from build123d import *

# Parameters (mm, degrees)
F1_DEPTH = 238.125
F3_DEPTH = 1.017


with BuildPart() as f1:
    # F0 (on Right) → F1 (new body, symmetric)
    with BuildSketch(Plane.YZ):
        Polygon((1.016, 17.526), (0, 17.526), (0, 12.446), (6.604, 12.446), (6.604, -12.446), (0, -12.446), (0, -17.526), (1.016, -17.526), (1.016, -13.462), (7.62, -13.462), (7.62, 13.462), (1.016, 13.462), align=None)
    extrude(amount=F1_DEPTH, both=True)

    # F2 (on face) → F3 (cut, through all)
    with BuildSketch(Plane.XZ.offset(-6.604)):
        with BuildLine():
            Line((-196.62013, 3.175), (-204.95387, 3.175))
            ThreePointArc((-204.95387, 3.175), (-208.12887, 0), (-204.95387, -3.175))
            Line((-204.95387, -3.175), (-196.62013, -3.175))
            ThreePointArc((-196.62013, -3.175), (-193.44513, 0), (-196.62013, 3.175))
        make_face()
        with BuildLine():
            ThreePointArc((-229.84587, 3.175), (-233.02087, 0), (-229.84587, -3.175))
            Line((-229.84587, -3.175), (-221.51213, -3.175))
            ThreePointArc((-221.51213, -3.175), (-218.33713, 0), (-221.51213, 3.175))
            Line((-221.51213, 3.175), (-229.84587, 3.175))
        make_face()
        with BuildLine():
            Line((-171.72813, 3.175), (-180.06187, 3.175))
            ThreePointArc((-180.06187, 3.175), (-183.23687, 0), (-180.06187, -3.175))
            Line((-180.06187, -3.175), (-171.72813, -3.175))
            ThreePointArc((-171.72813, -3.175), (-168.55313, 0), (-171.72813, 3.175))
        make_face()
        with BuildLine():
            Line((-146.83613, 3.175), (-155.16987, 3.175))
            ThreePointArc((-155.16987, 3.175), (-158.34487, 0), (-155.16987, -3.175))
            Line((-155.16987, -3.175), (-146.83613, -3.175))
            ThreePointArc((-146.83613, -3.175), (-143.66113, 0), (-146.83613, 3.175))
        make_face()
        with BuildLine():
            Line((-121.94413, 3.175), (-130.27787, 3.175))
            ThreePointArc((-130.27787, 3.175), (-133.45287, 0), (-130.27787, -3.175))
            Line((-130.27787, -3.175), (-121.94413, -3.175))
            ThreePointArc((-121.94413, -3.175), (-118.76913, 0), (-121.94413, 3.175))
        make_face()
        with BuildLine():
            Line((-97.05213, 3.175), (-105.38587, 3.175))
            ThreePointArc((-105.38587, 3.175), (-108.56087, 0), (-105.38587, -3.175))
            Line((-105.38587, -3.175), (-97.05213, -3.175))
            ThreePointArc((-97.05213, -3.175), (-93.87713, 0), (-97.05213, 3.175))
        make_face()
        with BuildLine():
            Line((-72.16013, 3.175), (-80.49387, 3.175))
            ThreePointArc((-80.49387, 3.175), (-83.66887, 0), (-80.49387, -3.175))
            Line((-80.49387, -3.175), (-72.16013, -3.175))
            ThreePointArc((-72.16013, -3.175), (-68.98513, 0), (-72.16013, 3.175))
        make_face()
        with BuildLine():
            Line((-47.26813, 3.175), (-55.60187, 3.175))
            ThreePointArc((-55.60187, 3.175), (-58.77687, 0), (-55.60187, -3.175))
            Line((-55.60187, -3.175), (-47.26813, -3.175))
            ThreePointArc((-47.26813, -3.175), (-44.09313, 0), (-47.26813, 3.175))
        make_face()
        with BuildLine():
            Line((-22.37613, 3.175), (-30.70987, 3.175))
            ThreePointArc((-30.70987, 3.175), (-33.88487, 0), (-30.70987, -3.175))
            Line((-30.70987, -3.175), (-22.37613, -3.175))
            ThreePointArc((-22.37613, -3.175), (-19.20113, 0), (-22.37613, 3.175))
        make_face()
        with BuildLine():
            Line((2.51587, 3.175), (-5.81787, 3.175))
            ThreePointArc((-5.81787, 3.175), (-8.99287, 0), (-5.81787, -3.175))
            Line((-5.81787, -3.175), (2.51587, -3.175))
            ThreePointArc((2.51587, -3.175), (5.69087, 0), (2.51587, 3.175))
        make_face()
        with BuildLine():
            Line((27.40787, 3.175), (19.07413, 3.175))
            ThreePointArc((19.07413, 3.175), (15.89913, 0), (19.07413, -3.175))
            Line((19.07413, -3.175), (27.40787, -3.175))
            ThreePointArc((27.40787, -3.175), (30.58287, 0), (27.40787, 3.175))
        make_face()
        with BuildLine():
            Line((52.29987, 3.175), (43.96613, 3.175))
            ThreePointArc((43.96613, 3.175), (40.79113, 0), (43.96613, -3.175))
            Line((43.96613, -3.175), (52.29987, -3.175))
            ThreePointArc((52.29987, -3.175), (55.47487, 0), (52.29987, 3.175))
        make_face()
        with BuildLine():
            Line((77.19187, 3.175), (68.85813, 3.175))
            ThreePointArc((68.85813, 3.175), (65.68313, 0), (68.85813, -3.175))
            Line((68.85813, -3.175), (77.19187, -3.175))
            ThreePointArc((77.19187, -3.175), (80.36687, 0), (77.19187, 3.175))
        make_face()
        with BuildLine():
            Line((102.08387, 3.175), (93.75013, 3.175))
            ThreePointArc((93.75013, 3.175), (90.57513, 0), (93.75013, -3.175))
            Line((93.75013, -3.175), (102.08387, -3.175))
            ThreePointArc((102.08387, -3.175), (105.25887, 0), (102.08387, 3.175))
        make_face()
        with BuildLine():
            Line((126.97587, 3.175), (118.64213, 3.175))
            ThreePointArc((118.64213, 3.175), (115.46713, 0), (118.64213, -3.175))
            Line((118.64213, -3.175), (126.97587, -3.175))
            ThreePointArc((126.97587, -3.175), (130.15087, 0), (126.97587, 3.175))
        make_face()
        with BuildLine():
            Line((151.86787, 3.175), (143.53413, 3.175))
            ThreePointArc((143.53413, 3.175), (140.35913, 0), (143.53413, -3.175))
            Line((143.53413, -3.175), (151.86787, -3.175))
            ThreePointArc((151.86787, -3.175), (155.04287, 0), (151.86787, 3.175))
        make_face()
        with BuildLine():
            Line((176.75987, 3.175), (168.42613, 3.175))
            ThreePointArc((168.42613, 3.175), (165.25113, 0), (168.42613, -3.175))
            Line((168.42613, -3.175), (176.75987, -3.175))
            ThreePointArc((176.75987, -3.175), (179.93487, 0), (176.75987, 3.175))
        make_face()
        with BuildLine():
            Line((201.65187, 3.175), (193.31813, 3.175))
            ThreePointArc((193.31813, 3.175), (190.14313, 0), (193.31813, -3.175))
            Line((193.31813, -3.175), (201.65187, -3.175))
            ThreePointArc((201.65187, -3.175), (204.82687, 0), (201.65187, 3.175))
        make_face()
        with BuildLine():
            Line((226.54387, 3.175), (218.21013, 3.175))
            ThreePointArc((218.21013, 3.175), (215.03513, 0), (218.21013, -3.175))
            Line((218.21013, -3.175), (226.54387, -3.175))
            ThreePointArc((226.54387, -3.175), (229.71887, 0), (226.54387, 3.175))
        make_face()
        with BuildLine():
            Line((251.43587, 3.175), (243.10213, 3.175))
            ThreePointArc((243.10213, 3.175), (239.92713, 0), (243.10213, -3.175))
            Line((243.10213, -3.175), (251.43587, -3.175))
            ThreePointArc((251.43587, -3.175), (254.61087, 0), (251.43587, 3.175))
        make_face()
    extrude(amount=-F3_DEPTH, mode=Mode.SUBTRACT)


solid = f1.part
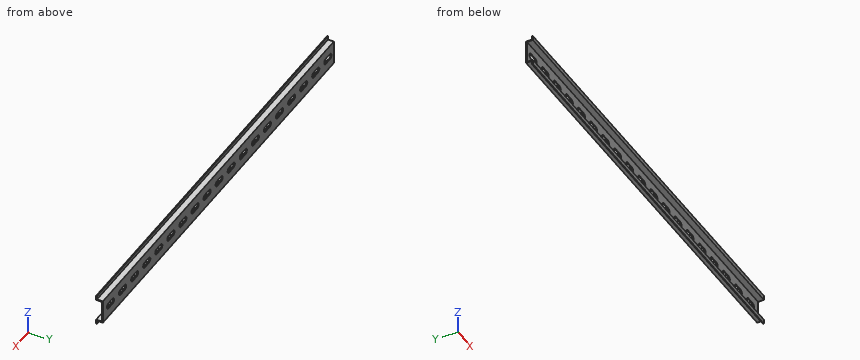
Source: CAD feature listing. Evaluate the final solid. Frame: model axes, mm. Round coordinates to 2 decimals unless told otherwise and drop trailing zeros. Loops run counter-clockwise (first coordinate to the right, second up) from the corner with the lowest first, then second, coordinate; pieces in that order, holes last.
Q1. Section A-A, the plane y = 4.5. Return loops of the section in (x, z) (3 decimals).
Q2. First-contact query: P1, Ø0.5, axis at x = 174.5, y = 7, coming from the +Z side; P2, Ø5, axis at x = 186, z = -1.5, coming from the -Y side; P3, Ø1.1, axis at x = 196.5, y = 7.5, coming from the -Z side. Flat tips, straight axial feed; report the tip coordinate or a pass-through.
Q3. Ray query, line 1 (Z direction, x = -208, y = 5); line 2 (Z direction, x = -171.5, y = 6.75); line 3 (Y direction, x = -152, z = -6). Return the intervals inside material, ascending.
Solutions:
1. outline: (-238.125, -13.462) - (238.125, -13.462) - (238.125, -12.446) - (-238.125, -12.446) - close; (-238.125, 12.446) - (238.125, 12.446) - (238.125, 13.462) - (-238.125, 13.462) - close
2. P1: stops at z = 13.46
2. P2: stops at y = 6.6
2. P3: stops at z = -13.46
3. line 1: z = -13.46 to -12.45, 12.45 to 13.46
3. line 2: z = -13.46 to -3.17, 3.17 to 13.46
3. line 3: y = 6.6 to 7.62
